```python
from build123d import *

# Parameters (mm, degrees)
EXTRUDE_1_DEPTH = 15
FILLET_1_R      = 2
FILLET_2_R      = 2.5
EXTRUDE_2_DEPTH = 362


# Read off the part's stored shape, not the designer's step: Отверстие с зазором M41
with BuildPart() as part:
    # Эскиз1 → Бобышка-Вытянуть1 (new body)
    with BuildSketch(Plane(origin=(0, 0, 0), x_dir=(1, 0, 0), z_dir=(0, 1, 0))):
        with BuildLine():
            Line((-22.5, -46.880166382), (-22.5, -45.768438907))
            ThreePointArc((-22.5, -45.768438907), (-17.354305588, -47.956522784), (-12, -49.568134926))
            Line((-12, -49.568134926), (-12, -58.568134926))
            Line((-12, -58.568134926), (12, -58.568134926))
            Line((12, -58.568134926), (12, -49.568134926))
            ThreePointArc((12, -49.568134926), (17.354305588, -47.956522784), (22.5, -45.768438907))
            Line((22.5, -45.768438907), (22.5, -46.880166382))
            ThreePointArc((22.5, -46.880166382), (17.834526239, -48.845979096), (13, -50.348783501))
            Line((13, -50.348783501), (13, -59.568134926))
            Line((13, -59.568134926), (-13, -59.568134926))
            Line((-13, -59.568134926), (-13, -50.348783501))
            ThreePointArc((-13, -50.348783501), (-17.834526239, -48.845979096), (-22.5, -46.880166382))
        make_face()
    extrude(amount=EXTRUDE_1_DEPTH)

    # Скругление1
    fillet_1_edges = [part.edges().sort_by_distance(p)[0] for p in [
        (-13, 7.5, 50.348783501),
        (13, 7.5, 50.348783501),
        (12, 7.5, 58.568134926),
        (-12, 7.5, 58.568134926),
    ]]
    fillet(fillet_1_edges, radius=FILLET_1_R)

    # Скругление2
    fillet_2_edges = [part.edges().sort_by_distance(p)[0] for p in [
        (-12, 7.5, 49.568134926),
        (-13, 7.5, 59.568134926),
        (13, 7.5, 59.568134926),
        (12, 7.5, 49.568134926),
    ]]
    fillet(fillet_2_edges, radius=FILLET_2_R)

    # Отверстие с зазором M41 outline → Отверстие с зазором M41 (revolve, cut)
    with BuildSketch(Plane(origin=(0, 8, 0), x_dir=(0.9280125149960182, 0, -0.37254901960784303), z_dir=(0, -1, 0))):
        Polygon((2.25, 52.000021479), (2.25, 51.975), (2.275021479, 52.000021479), align=None)
        Polygon((2.25, 50.950316764), (2.25, 51.975), (2.25, 52.000021479), (0, 52.000021479), (0, 50.950316764), align=None)
    revolve(axis=Axis((0, 8, 0), (0.37254901960784303, 0, 0.9280125149960182)), mode=Mode.SUBTRACT)

    # Hole Wizard M41 2 outline → Hole Wizard M41 2 (revolve, cut)
    with BuildSketch(Plane(origin=(0, 8, 0), x_dir=(0.9280125149960182, 0, 0.37254901960784303), z_dir=(0, 1, 0))):
        Polygon((2.25, -52.000019282), (2.25, -51.975), (2.25, -50.950316764), (0, -50.950316764), (0, -52.000019282), align=None)
        Polygon((2.275019282, -52.000019282), (2.249998249, -51.974998249), (2.25, -52.000019282), align=None)
    revolve(axis=Axis((0, 8, 0), (0.37254901960784303, 0, -0.9280125149960182)), mode=Mode.SUBTRACT)

    # Эскиз3 → Бобышка-Вытянуть2 (add)
    with BuildSketch(Plane.XZ):
        with BuildLine():
            Line((12, 56.568134926), (12, 51.497572758))
            ThreePointArc((12, 51.497572758), (12.507021672, 49.988255899), (13.822429907, 49.091144125))
            ThreePointArc((13.822429907, 49.091144125), (18.237045294, 47.627829878), (22.5, 45.768438907))
            Line((22.5, 45.768438907), (22.5, 46.880166382))
            ThreePointArc((22.5, 46.880166382), (18.536030559, 48.584108216), (14.444444444, 49.953558679))
            ThreePointArc((14.444444444, 49.953558679), (13.401389492, 50.672998972), (13, 51.874849397))
            Line((13, 51.874849397), (13, 57.068134926))
            ThreePointArc((13, 57.068134926), (12.267766953, 58.835901879), (10.5, 59.568134926))
            Line((10.5, 59.568134926), (-10.5, 59.568134926))
            ThreePointArc((-10.5, 59.568134926), (-12.267766953, 58.835901879), (-13, 57.068134926))
            Line((-13, 57.068134926), (-13, 51.874849397))
            ThreePointArc((-13, 51.874849397), (-13.401389492, 50.672998972), (-14.444444444, 49.953558679))
            ThreePointArc((-14.444444444, 49.953558679), (-18.536030559, 48.584108216), (-22.5, 46.880166382))
            Line((-22.5, 46.880166382), (-22.5, 45.768438907))
            ThreePointArc((-22.5, 45.768438907), (-18.237045294, 47.627829878), (-13.822429907, 49.091144125))
            ThreePointArc((-13.822429907, 49.091144125), (-12.507021672, 49.988255899), (-12, 51.497572758))
            Line((-12, 51.497572758), (-12, 56.568134926))
            ThreePointArc((-12, 56.568134926), (-11.414213562, 57.982348488), (-10, 58.568134926))
            Line((-10, 58.568134926), (10, 58.568134926))
            ThreePointArc((10, 58.568134926), (11.414213562, 57.982348488), (12, 56.568134926))
        make_face()
    extrude(amount=EXTRUDE_2_DEPTH)


solid = part.part
```
Read the model definition and answer for the solid it produces. Units are mm, in the model's axes. Coordinates: 2 decimals unless noted, no trailing zeros. Loops run counter-clockwise (first coordinate to the right, second up) from the corner with the lowest first, then second, coordinate; pieces in that order, holes last.
(1) The mould has two halves that part along X. Classify faces 1 (the face through (0, -171, 59.568)), 2 (the face through (0, -171, 58.568)): released by +X, released by -X, zero draft, split by the parting line, or undercut.
Solution:
face 1: zero draft
face 2: undercut
(2) The part is cut by section A-A (y = -128). Determine the outline of the cut face in (x, z), and give its area (3 significant figures).
Solution:
outline: (-22.5, 45.77) arc R51 cw to (-13.82, 49.09) arc R2.5 ccw to (-12, 51.5) - (-12, 56.57) arc R2 cw to (-10, 58.57) - (10, 58.57) arc R2 cw to (12, 56.57) - (12, 51.5) arc R2.5 ccw to (13.82, 49.09) arc R51 cw to (22.5, 45.77) - (22.5, 46.88) arc R52 ccw to (14.44, 49.95) arc R2 cw to (13, 51.87) - (13, 57.07) arc R2.5 ccw to (10.5, 59.57) - (-10.5, 59.57) arc R2.5 ccw to (-13, 57.07) - (-13, 51.87) arc R2 cw to (-14.44, 49.95) arc R52 ccw to (-22.5, 46.88) - close
area: 63.0 mm2
(3) Consider line 1 along X through (y, z) = (-111.5, 56.25); line 2 along Z through (x, y) = (-1.5, -167.5); line 3 along X through (y, z) = (-24, 50.5). Determine where each line is inside the solid, lowest interval first.
Solution:
line 1: x = -13 to -12, 12 to 13
line 2: z = 58.57 to 59.57
line 3: x = -13.55 to -12.21, 12.21 to 13.55
(4) The part is cut by section B-B (x = -2). Determine the outline of the cut face in (y, z), and give its area (3 significant figures).
Solution:
outline: (-362, 58.57) - (15, 58.57) - (15, 59.57) - (-362, 59.57) - close
area: 377 mm2
(5) Flat-ended cylindrical pins translate along their axes: pin 1 Ø10 at (x, y) = (-17.5, -74) entering from +Z; pin 2 Ø3 at (x, z) = (11.5, 50) entering from -Y; pin 3 Ø16 at (x, y) = (-1.5, -240.5) entering from -Z; pin 4 Ø1.6 at (y, z) = (-180, 53.5) entering from -X. Find the tip coordinate at first contact, or state that the pin passes through.
Solution:
pin 1: stops at z = 58.57
pin 2: stops at y = -362
pin 3: stops at z = 58.57
pin 4: stops at x = -13
